Autodesk Inventor part; units mm, degrees
ref_plane "YZ Plane" through (0, 0, 0) normal (1, 0, 0) x (0, 1, 0)
ref_plane "XZ Plane" through (0, 0, 0) normal (0, 1, 0) x (-1, 0, 0)
ref_plane "XY Plane" through (0, 0, 0) normal (0, 0, 1) x (1, 0, 0)
sketch "Sketch1" plane through (0, 0, 0) normal (0, 1, 0) x (-1, 0, 0)
  circle A0 centre (25, 36.3) radius 2.5
  circle A1 centre (33, 49.9) radius 2.5
  line L0 (15, 0) -> (15, 15)
  line L1 (15, 15) -> (0, 15)
  line L2 (0, 15) -> (0, 80)
  line L3 (0, 80) -> (41, 80)
  line L4 (41, 80) -> (41, 0)
  line L5 (15, 0) -> (41, 0)
  circle A2 centre (25, 36.3) radius 7.5 construction
  circle A3 centre (33, 49.9) radius 7.5 construction
  point P0 (0, 0)
  dimension "d0" = 5
  dimension "d1" = 15
  dimension "d2" = 25
  dimension "d3" = 21.3
  dimension "d4" = 8
  dimension "d5" = 13.6
  dimension "d12" = 15
  dimension "d46" = 80
  dimension "d47" = 41
extrude "Extrusion1" add sketch "Sketch1" along normal blind 3
sketch "Sketch2" plane through (0, 3, 0) normal (0, 1, 0) x (1, 0, 0)
  line L0 (-41, 0) -> (-41, -80)
  line L1 (-41, -80) -> (0, -80)
  line L2 (0, -80) -> (0, -15)
  line L3 (0, -15) -> (-15, -15)
  line L4 (-15, -15) -> (-15, 0)
  line L5 (-15, 0) -> (-41, 0)
  circle A0 centre (-33, -49.9) radius 2.5
  circle A1 centre (-25, -36.3) radius 2.5
  line L6 (-15, -15) -> (-15, 0)
  line L7 (-15, -15) -> (-15, -80)
  line L8 (-15, -15) -> (-41, -15)
  line L9 (-41, 0) -> (-41, -80)
  point P0 (0, 0)
extrude "Extrusion2" add sketch "Sketch2" along normal blind 3 contours L5 L4 L8 L0 | L3 L2 L1 L7
sketch "Sketch3" plane through (0, 3, 0) normal (0, 1, 0) x (1, 0, 0)
  circle A0 centre (-25, -36.3) radius 2.5
  circle A1 centre (-33, -49.9) radius 2.5
  line L0 (-15, -80) -> (-15, -15)
  line L1 (-15, -15) -> (-41, -15)
  line L2 (-41, -15) -> (-41, -80)
  line L3 (-41, -80) -> (-15, -80)
  circle A2 centre (-25, -36.3) radius 2.5
  circle A3 centre (-25, -36.3) radius 8.5
  circle A4 centre (-33, -49.9) radius 2.5
  circle A5 centre (-33, -49.9) radius 8.5
  line L4 (-31.8739, -31.3) -> (-41, -31.3)
  line L5 (-41, 0) -> (-41, -80)
  line L6 (-33, -41.4) -> (-41, -41.4)
  line L7 (-38.3753, -56.4846) -> (-41, -56.4846)
  line L8 (-29, -57.4) -> (-29, -80)
  line L9 (-41, -80) -> (0, -80)
  point P0 (0, 0)
  point P1 (-31.727, -41.4959)
  dimension "d15" = 17
  dimension "d16" = 5
  dimension "d19" = 12
extrude "Extrusion3" add sketch "Sketch3" along normal blind 21 contours L3 L2 L7 A5 L8 | L4 A3 A5 L6 L2
fillet "Fillet1" radius 1 8 edges at (-31.8739, 13.5, 31.3) (-31.727, 13.5, 41.4959) (-41, 13.5, 41.4) (-41, 13.5, 31.3) (-41, 13.5, 56.4846) (-29, 13.5, 57.4) (-29, 13.5, 80) (-38.3753, 13.5, 56.4846)
chamfer "Chamfer1" distance 10 angle 45 1 edges at (-41, 12, 80)
sketch "Sketch4" plane through (0, 24, 0) normal (0, 1, 0) x (1, 0, 0)
  line L0 (-31, -80) -> (-41, -70)
  line L1 (-31, -80) -> (-30, -80)
  arc A0 (-30, -80) -> (-29, -79) centre (-30, -79) ccw
  line L2 (-29, -79) -> (-29, -58.9139)
  arc A1 (-29, -58.9139) -> (-30.3158, -57.965) centre (-30, -58.9139) ccw
  arc A2 (-38.1184, -56.6862) -> (-30.3158, -57.965) centre (-33, -49.9) ccw
  arc A3 (-38.1184, -56.6862) -> (-38.7205, -56.4846) centre (-38.7205, -57.4846) ccw
  line L3 (-38.7205, -56.4846) -> (-40, -56.4846)
  arc A4 (-40, -56.4846) -> (-41, -57.4846) centre (-40, -57.4846) ccw
  line L4 (-41, -57.4846) -> (-41, -70)
  arc A5 (-40, -31.3) -> (-41, -32.3) centre (-40, -32.3) ccw
  line L5 (-41, -32.3) -> (-41, -40.4)
  arc A6 (-41, -40.4) -> (-40, -41.4) centre (-40, -40.4) ccw
  line L6 (-40, -41.4) -> (-33.5697, -41.4)
  arc A7 (-33.5697, -41.4) -> (-32.6676, -39.9684) centre (-33.5697, -40.4) ccw
  arc A8 (-32.7098, -32.7211) -> (-32.6676, -39.9684) centre (-25, -36.3) ccw
  arc A9 (-32.7098, -32.7211) -> (-33.6168, -31.3) centre (-33.6168, -32.3) ccw
  line L7 (-33.6168, -31.3) -> (-40, -31.3)
  point P0 (0, 0)
  point P1 (-37, -36)
  point P2 (-37, -66)
  dimension "d24" = 4
  dimension "d25" = 36
  dimension "d26" = 30
hole "Hole1" at (-37, 24, 36) at (-37, 24, 66) direction (0, -1, 0) diameter 2.8 depth 10 tip angle 118
sketch "Sketch5" plane through (0, 0, 0) normal (0, -1, 0) x (1, 0, 0)
  line L0 (-41, 70) -> (-31, 80)
  line L1 (-41, 0) -> (-41, 70)
  line L2 (-15, 0) -> (-41, 0)
  line L3 (-15, 15) -> (-15, 0)
  line L4 (0, 15) -> (-15, 15)
  line L5 (0, 80) -> (0, 15)
  line L6 (-31, 80) -> (0, 80)
  circle A0 centre (-33, 49.9) radius 2.5
  circle A1 centre (-25, 36.3) radius 2.5
  point P0 (0, 0)
  point P1 (-31, 7.5)
  point P2 (-7.5, 25)
  point P3 (-7.5, 65)
  dimension "d34" = 7.5
  dimension "d35" = 7.5
  dimension "d36" = 10
  dimension "d37" = 15
  dimension "d38" = 40
hole "Hole2" at (-31, 0, 7.5) at (-7.5, 0, 25) at (-7.5, 0, 65) direction (0, 1, 0) diameter 3.6 end through all counterbore diameter 6.5 counterbore depth 3.4
sketch "Sketch6" plane through (0, 0, 0) normal (0, -1, 0) x (1, 0, 0)
  circle A0 centre (-7.5, 25) radius 3.25
  circle A1 centre (-31, 7.5) radius 3.25
  circle A2 centre (-7.5, 65) radius 3.25
  line L0 (-41, 70) -> (-31, 80)
  line L1 (-41, 0) -> (-41, 70)
  line L2 (-15, 0) -> (-41, 0)
  line L3 (-15, 15) -> (-15, 0)
  line L4 (0, 15) -> (-15, 15)
  line L5 (0, 80) -> (0, 15)
  line L6 (-31, 80) -> (0, 80)
  circle A3 centre (-33, 49.9) radius 2.5
  circle A4 centre (-25, 36.3) radius 2.5
  point P0 (0, 0)
  point P1 (-23, 13)
  point P2 (-23, 28)
  dimension "d48" = 15
  dimension "d49" = 8
  dimension "d50" = 13
hole "Hole3" at (-23, 0, 13) at (-23, 0, 28) direction (0, 1, 0) diameter 2.8 end through all
properties part number "Alpha Idler Assembly" material "ABS Plastic"
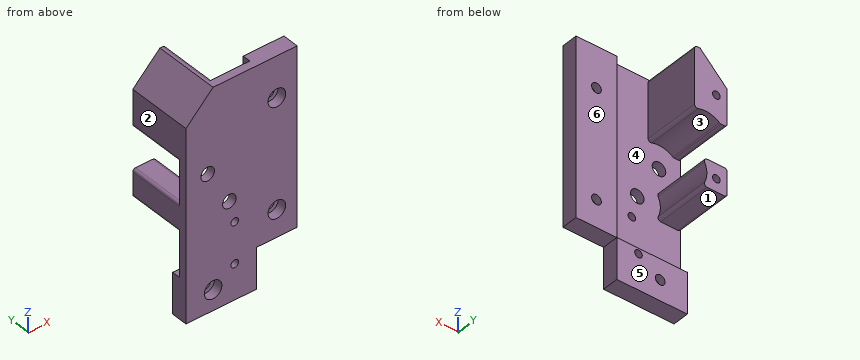
Input: part model. Units: mm. Frame: model coordinates. Face numbers are marked on the shaded views. A direction names the side the tool comes from. Coordinates: 2 decimals unless noted, no trailing zeros. Order: outer loops, then holes, each group sorted by start corner. A loop starts at its lowest first (then second) coordinate and runs counter-clockwise, first axis right, second up. Notation, with made-up numbers: M 1.25,3.25 L 27.25,3.25 A27 cw 27.25,36.25 Z; hole C 39,60 d4. An arc over 180 degrees is marked long. Answer in a Markdown table with one row per item.
(1) Section query B-B, the plane z = 72. Output: boundary loops of the cut face in (x, y), plus the area to 3 significant figures.
Numbers:
| item | result |
|---|---|
| outline | M -39,0 L 0,0 L 0,6 L -15,6 L -15,3 L -29,3 L -29,24 L -39,24 Z |
| area | 372 mm^2 |
(2) Section query A-A, the plane z = 25. Output: boundary loops of the cut face in (x, y).
Numbers:
| item | result |
|---|---|
| outline | M -41,0 L -10.75,0 L -10.75,3.4 L -9.3,3.4 L -9.3,6 L -15,6 L -15,3 L -41,3 Z; M -5.7,3.4 L -4.25,3.4 L -4.25,0 L 0,0 L 0,6 L -5.7,6 Z |
(3) Material intervals for line 1 (X direction, y = 5.5, z = 65); line 2 (Z direction, x = -7.5, y = 0.7); line 3 (Z direction, x = -23, y = 3.25), sorted ascending. Write a range as [from, to].
Numbers:
| item | result |
|---|---|
| line 1 | x = [-41, -29], [-15, -9.3], [-5.7, 0] |
| line 2 | z = [15, 21.75], [28.25, 61.75], [68.25, 80] |
| line 3 | z = [0, 11.6], [14.4, 15] |
(4) Section query D-D, the plane z = 13. Output: boundary loops of the cut face in (x, y), plus the area to 3 significant figures.
Numbers:
| item | result |
|---|---|
| outline | M -41,0 L -24.4,0 L -24.4,6 L -41,6 Z; M -21.6,0 L -15,0 L -15,6 L -21.6,6 Z |
| area | 139 mm^2 |
(5) Access query for the marked faces 4, 5 and 6. Directions: +Z, -Z, +X, -X, +Y, -Y. A direction counts if a zero-diameter tool reaches every point of the face in a straight line with its end or side. Return the directions, or none.
Numbers:
| item | result |
|---|---|
| face 4 | +Y |
| face 5 | -Z, +X, -X, +Y |
| face 6 | +Z, -Z, +X, +Y |
(6) Contact query for flat-ended pins moving along their axis: pin 1 Ø3 at (x, z) = (-26.5, 61.5) entering from +Y; pin 2 Ø5 at (x, z) = (-7.5, 65) entering from -Y; pin 3 Ø4.5 at (x, z) = (-25, 36.3) entering from +Y; pin 4 Ø2 at (y, z) = (3.5, 11.5) entering from +X. Output: stop coordinate, or through.
Numbers:
| item | result |
|---|---|
| pin 1 | stops at y = 3 |
| pin 2 | stops at y = 3.4 |
| pin 3 | passes through |
| pin 4 | stops at x = -15 |
(7) Section query C-C, the plane y = 21. Give the number of separate pieces and of enclosed holes in the cut face, plus the area to 3 significant figures.
Numbers:
| item | result |
|---|---|
| separate pieces | 2 |
| enclosed holes | 2 |
| area | 285 mm^2 |
(8) Draft query along X for the marked faces 1, 2 and 3. Return one class per face: pulls with the +X half, pulls with the -X half, needs draft (parallel to the pull), parting line crosses it, or undercut.
Numbers:
| item | result |
|---|---|
| face 1 | needs draft |
| face 2 | pulls with the -X half |
| face 3 | undercut |
